Read the model definition and answer for the solid it produces. Units are mm, in the model's axes. A direction names the side the tool comes from. Coordinates: 2 decimals unless noted, no trailing zeros. Write each loop counter-clockwise with the first axis right and the second up, starting at its lowest first coordinate (ties: lowest second). Pieces come first, ordered by that corner, then holes. Notation, with made-up numbers: (14.25, -26.5) -> (70.25, -26.5) arc R7 ccw to (70.25, -20.5) -> close; hole circle Ø7 at (-14.5, -39.5). An arc over 180 degrees is marked (long way). Answer in a Markdown table with one row per item. Add a question column.
Item 1: Which of the six approach directions +Z, -Z, +X, -X, +Y, -Y give full straight-line access (tool end or side, diameter ignored) to faces 5 (the face through (15, 37, 2)), 6 (the face through (15, 83, 1)), 7 (the face through (22, 60, 1))?
Item 2: Section D-D on x = 2.5 is taken. Write down the section's boundary in (y, z).
Item 3: Section C-C on y = 49 is taken. Write down the section's boundary in (x, z).
Item 4: Given pin 1 Ø0.6 at (y, z) = (72.5, 0.5) entering from +X, flat-ended and moving along its own axis, determine where the tip first touches the part or whether it passes through.
Item 5: Section B-B on z = 1.1 is taken. Write down the section's boundary in (x, y), then the cut area to 3 significant figures.
Item 6: For a pull along X with two mould halves and no side action, classify faces 1 (the face through (13.5, 74, 1)), 2 (the face through (8, 61, 1)), 3 (the face through (15, 94, 1)), 4 (the face through (16.5, 74, 1)) as +X half, -X half, draft (parallel to the pull), parting line (faces both ways), or undercut.
Item 7: Section A-A on y = 67 is taken. Write down the section's boundary in (x, z), then the cut area to 3 significant figures.
Item 8: Straight lines are drawn through the part: line 1 (X direction, y = 77, z = 1.5); line 2 (X direction, y = 58.5, z = 1.35); line 3 (Y direction, x = 5.75, z = 1.7). For each, find the intervals that lie inside material, in ascending order. Write a range as from..to.
```python
from build123d import *

# Parameters (mm, degrees)
COPYSKETCH_W = 3
COPYSKETCH_H = 17
PAD_DEPTH    = 2


with BuildPart() as part:
    # CopySketch → Pad (new body)
    with BuildSketch(Plane.XY):
        with BuildLine():
            Line((0, 0), (30, 0))
            Line((30, 0), (30, 20))
            Line((30, 20), (29.5, 20))
            ThreePointArc((22, 27.5), (24.196699, 22.196699), (29.5, 20))
            Line((22, 27.5), (22, 94))
            Line((22, 94), (8, 94))
            Line((8, 94), (8, 27.5))
            ThreePointArc((0.5, 20), (5.803301, 22.196699), (8, 27.5))
            Line((0, 20), (0.5, 20))
            Line((0, 20), (0, 0))
        make_face()
        with Locations((15, 74.5)):
            Rectangle(COPYSKETCH_W, COPYSKETCH_H, mode=Mode.SUBTRACT)
    extrude(amount=PAD_DEPTH)


solid = part.part
```
Results below:
| question | item | result |
|---|---|---|
| 1 | face 5 | +Z, +X, -X, +Y, -Y |
| 1 | face 6 | +Z, -Z |
| 1 | face 7 | +Z, -Z, +X, +Y |
| 2 | outline | (0, 0) -> (20.27, 0) -> (20.27, 2) -> (0, 2) -> close |
| 3 | outline | (8, 0) -> (22, 0) -> (22, 2) -> (8, 2) -> close |
| 4 | pin 1 | stops at x = 22 |
| 5 | outline | (0, 0) -> (30, 0) -> (30, 20) -> (29.5, 20) arc R7.5 cw to (22, 27.5) -> (22, 94) -> (8, 94) -> (8, 27.5) arc R7.5 cw to (0.5, 20) -> (0, 20) -> close; hole (13.5, 66) -> (16.5, 66) -> (16.5, 83) -> (13.5, 83) -> close |
| 5 | area | 1,610 mm2 |
| 6 | face 1 | undercut |
| 6 | face 2 | -X half |
| 6 | face 3 | draft |
| 6 | face 4 | undercut |
| 7 | outline | (8, 0) -> (13.5, 0) -> (13.5, 2) -> (8, 2) -> close; (16.5, 0) -> (22, 0) -> (22, 2) -> (16.5, 2) -> close |
| 7 | area | 22.0 mm2 |
| 8 | line 1 | x = 8..13.5, 16.5..22 |
| 8 | line 2 | x = 8..22 |
| 8 | line 3 | y = 0..22.14 |
